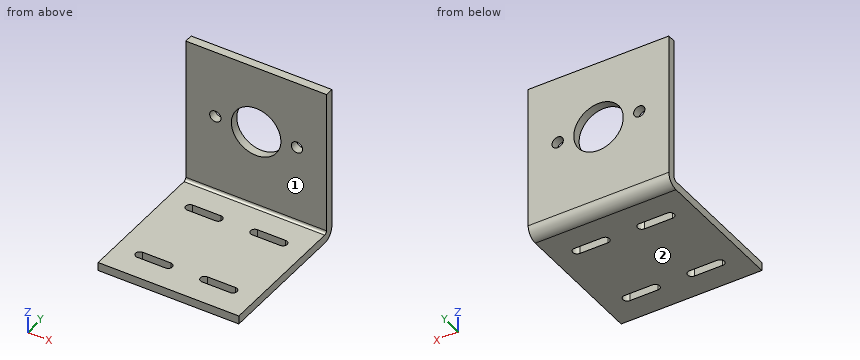
from build123d import *

# Parameters (mm, degrees)
SKETCH1_W           = 50
SKETCH1_H           = 52
BOSS_EXTRUDE1_DEPTH = 3
SKETCH2_W           = 50
SKETCH2_H           = 3
BOSS_EXTRUDE2_DEPTH = 52
FILLET1_R           = 4
FILLET2_R           = 1
CUT_EXTRUDE1_REACH  = 92.714
SKETCH3_R           = 2
SKETCH3_R_2         = 8.8
CUT_EXTRUDE2_REACH  = 90.927


with BuildPart() as part:
    # Sketch1 → Boss-Extrude1 (new body)
    with BuildSketch(Plane.XY):
        with Locations((25, 26)):
            Rectangle(SKETCH1_W, SKETCH1_H)
    extrude(amount=BOSS_EXTRUDE1_DEPTH)

    # Sketch2 → Boss-Extrude2 (add)
    with BuildSketch(Plane.XY.offset(3)):
        with Locations((25, 50.5)):
            Rectangle(SKETCH2_W, SKETCH2_H)
    extrude(amount=BOSS_EXTRUDE2_DEPTH)

    # Fillet1
    fillet1_edges = [part.edges().sort_by_distance(p)[0] for p in [
        (25, 52, 0),
    ]]
    fillet(fillet1_edges, radius=FILLET1_R)

    # Fillet2
    fillet2_edges = [part.edges().sort_by_distance(p)[0] for p in [
        (25, 49, 3),
    ]]
    fillet(fillet2_edges, radius=FILLET2_R)

    # Sketch3 → Cut-Extrude1 (cut, up to next)
    with BuildSketch(Plane(origin=(0, 52, 0), x_dir=(1, 0, 0), z_dir=(0, 1, 0)), mode=Mode.PRIVATE) as cut_extrude1_sk1:
        with Locations(Location((10.5, -31, 0), (0, 0, 270))):
            Circle(SKETCH3_R)
    cut_extrude1_tool1 = extrude(cut_extrude1_sk1.sketch, amount=-CUT_EXTRUDE1_REACH, mode=Mode.PRIVATE) & part.part
    # Sketch3 → Cut-Extrude1 (cut, up to next)
    with BuildSketch(Plane(origin=(0, 52, 0), x_dir=(1, 0, 0), z_dir=(0, 1, 0)), mode=Mode.PRIVATE) as cut_extrude1_sk2:
        with Locations(Location((39.5, -31, 0), (0, 0, 270))):
            Circle(SKETCH3_R)
    cut_extrude1_tool2 = extrude(cut_extrude1_sk2.sketch, amount=-CUT_EXTRUDE1_REACH, mode=Mode.PRIVATE) & part.part
    # Sketch3 → Cut-Extrude1 (cut, up to next)
    with BuildSketch(Plane(origin=(0, 52, 0), x_dir=(1, 0, 0), z_dir=(0, 1, 0)), mode=Mode.PRIVATE) as cut_extrude1_sk3:
        with Locations(Location((25, -31, 0), (0, 0, 270))):
            Circle(SKETCH3_R_2)
    cut_extrude1_tool3 = extrude(cut_extrude1_sk3.sketch, amount=-CUT_EXTRUDE1_REACH, mode=Mode.PRIVATE) & part.part
    add(cut_extrude1_tool1.solids().sort_by_distance((10.5, 52, 31))[0], mode=Mode.SUBTRACT)
    add(cut_extrude1_tool2.solids().sort_by_distance((39.5, 52, 31))[0], mode=Mode.SUBTRACT)
    add(cut_extrude1_tool3.solids().sort_by_distance((25, 52, 31))[0], mode=Mode.SUBTRACT)

    # Sketch6 → Cut-Extrude2 (cut, up to next)
    with BuildSketch(Plane.XY.offset(3), mode=Mode.PRIVATE) as cut_extrude2_sk1:
        with BuildLine():
            Line((8.5, 39.5), (18.5, 39.5))
            ThreePointArc((18.5, 39.5), (20, 38), (18.5, 36.5))
            Line((18.5, 36.5), (8.5, 36.5))
            ThreePointArc((8.5, 36.5), (7, 38), (8.5, 39.5))
        make_face()
    cut_extrude2_tool1 = extrude(cut_extrude2_sk1.sketch, amount=-CUT_EXTRUDE2_REACH, mode=Mode.PRIVATE) & part.part
    # Sketch6 → Cut-Extrude2 (cut, up to next)
    with BuildSketch(Plane.XY.offset(3), mode=Mode.PRIVATE) as cut_extrude2_sk2:
        with BuildLine():
            Line((41.5, 39.5), (31.5, 39.5))
            ThreePointArc((31.5, 39.5), (30, 38), (31.5, 36.5))
            Line((31.5, 36.5), (41.5, 36.5))
            ThreePointArc((41.5, 36.5), (43, 38), (41.5, 39.5))
        make_face()
    cut_extrude2_tool2 = extrude(cut_extrude2_sk2.sketch, amount=-CUT_EXTRUDE2_REACH, mode=Mode.PRIVATE) & part.part
    # Sketch6 → Cut-Extrude2 (cut, up to next)
    with BuildSketch(Plane.XY.offset(3), mode=Mode.PRIVATE) as cut_extrude2_sk3:
        with BuildLine():
            Line((8.5, 8.5), (18.5, 8.5))
            ThreePointArc((18.5, 8.5), (20, 10), (18.5, 11.5))
            Line((18.5, 11.5), (8.5, 11.5))
            ThreePointArc((8.5, 11.5), (7, 10), (8.5, 8.5))
        make_face()
    cut_extrude2_tool3 = extrude(cut_extrude2_sk3.sketch, amount=-CUT_EXTRUDE2_REACH, mode=Mode.PRIVATE) & part.part
    # Sketch6 → Cut-Extrude2 (cut, up to next)
    with BuildSketch(Plane.XY.offset(3), mode=Mode.PRIVATE) as cut_extrude2_sk4:
        with BuildLine():
            Line((41.5, 8.5), (31.5, 8.5))
            ThreePointArc((31.5, 8.5), (30, 10), (31.5, 11.5))
            Line((31.5, 11.5), (41.5, 11.5))
            ThreePointArc((41.5, 11.5), (43, 10), (41.5, 8.5))
        make_face()
    cut_extrude2_tool4 = extrude(cut_extrude2_sk4.sketch, amount=-CUT_EXTRUDE2_REACH, mode=Mode.PRIVATE) & part.part
    add(cut_extrude2_tool1.solids().sort_by_distance((13.5, 38, 3))[0], mode=Mode.SUBTRACT)
    add(cut_extrude2_tool2.solids().sort_by_distance((36.5, 38, 3))[0], mode=Mode.SUBTRACT)
    add(cut_extrude2_tool3.solids().sort_by_distance((13.5, 10, 3))[0], mode=Mode.SUBTRACT)
    add(cut_extrude2_tool4.solids().sort_by_distance((36.5, 10, 3))[0], mode=Mode.SUBTRACT)


solid = part.part
The listing builds one solid part. Answer for the finished solid, in the listing's coordinates (mm). Face numbers are marked on the shaded views. A direction names the side the tool comes from. Give positions to 0.01 mm unless a question says otherwise; leave off trailing zeros. Loops run counter-clockwise (first coordinate to the right, second up) from the corner with the lowest first, then second, coordinate; pieces in that order, holes last. Notation, with made-up numbers: (-36, 55) - (-16, 55) arc R29 cw to (-16, 92) - close; hole circle Ø5 at (-11, 46). An arc over 180 degrees is marked (long way). Answer as a JSON object with one key per item and string values.
1. A cutting plane is placed at B-B (z = 31). Write down the section's boundary in (x, y), then the cut area to 3 significant figures.
Determined:
{"outline": "(0, 49) - (8.5, 49) - (8.5, 52) - (0, 52) - close; (12.5, 49) - (16.2, 49) - (16.2, 52) - (12.5, 52) - close; (33.8, 49) - (37.5, 49) - (37.5, 52) - (33.8, 52) - close; (41.5, 49) - (50, 49) - (50, 52) - (41.5, 52) - close", "area": "73.2 mm²"}
2. A cutting plane is placed at C-C (y = 38). Write down the section's boundary in (x, z).
Determined:
{"outline": "(0, 0) - (7, 0) - (7, 3) - (0, 3) - close; (20, 0) - (30, 0) - (30, 3) - (20, 3) - close; (43, 0) - (50, 0) - (50, 3) - (43, 3) - close"}
3. A cutting plane is placed at A-A (x = 10.5). Write down the section's boundary in (y, z), then the cut area to 3 significant figures.
Determined:
{"outline": "(0, 0) - (8.5, 0) - (8.5, 3) - (0, 3) - close; (11.5, 0) - (36.5, 0) - (36.5, 3) - (11.5, 3) - close; (39.5, 0) - (48, 0) arc R4 ccw to (52, 4) - (52, 29) - (49, 29) - (49, 4) arc R1 cw to (48, 3) - (39.5, 3) - close; (49, 33) - (52, 33) - (52, 55) - (49, 55) - close", "area": "279 mm²"}
4. A cutting plane is placed at D-D (x = 25). Write down the section's boundary in (y, z), then the cut area to 3 significant figures.
Determined:
{"outline": "(0, 0) - (48, 0) arc R4 ccw to (52, 4) - (52, 22.2) - (49, 22.2) - (49, 4) arc R1 cw to (48, 3) - (0, 3) - close; (49, 39.8) - (52, 39.8) - (52, 55) - (49, 55) - close", "area": "256 mm²"}
5. Flat-ended cylindrical pins translate along their axes: pin 1 Ø8 at (y, z) = (36.5, 7.5) entering from -X; pin 2 Ø23 at (x, z) = (25, 31) entering from -Y; pin 3 Ø3.5 at (x, z) = (15, 1.5) entering from +Y; pin 4 Ø2.5 at (x, z) = (37.5, 1.5) entering from +Y. Find the tip coordinate at first contact, or state that the pin passes through.
Determined:
{"pin 1": "through", "pin 2": "y = 49", "pin 3": "y = 51.93", "pin 4": "y = 51.8"}
6. For the marked faces 1 and 2, determine the directions among +Z, -Z, +X, -X, +Y, -Y from which every point of the face is accessible in a straight line to the end or side of a thin tool.
Determined:
{"face 1": "+Z, +X, -X, -Y", "face 2": "-Z, +X, -X, +Y, -Y"}
7. Find the intervals of material crossed by L1, parallel to X at y = 50.6, z = 31; L2, parallel to Y at x = 30, z = 14; L3, parallel to Z at x = 32, y = 27.5, in increasing order. Write a range as [from, to].
Determined:
{"L1": "[0, 8.5], [12.5, 16.2], [33.8, 37.5], [41.5, 50]", "L2": "[49, 52]", "L3": "[0, 3]"}
